```python
from build123d import *

# Parameters (mm, degrees)
SKETCH1_R               = 0.8
BOSS_EXTRUDE1_DEPTH     = 0.75
SKETCH2_R               = 0.8
BOSS_EXTRUDE2_DEPTH     = 2.5
CHAMFER1_SIZE           = 1.625
CUT_EXTRUDE1_DEPTH      = 24.451236904
CUT_EXTRUDE1_DEPTH_BACK = 24.451236904
SKETCH3_W               = 10.5
SKETCH3_H               = 2


with BuildPart() as part:
    # Sketch1 → Boss-Extrude1 (new, symmetric)
    with BuildSketch(Plane(origin=(0, 0, 0), x_dir=(1, 0, 0), z_dir=(0, 1, 0))):
        with BuildLine():
            ThreePointArc((1.600460999, 1.920553199), (-1.920553199, 1.600460999), (-1.600460999, -1.920553199))
            ThreePointArc((-1.600460999, -1.920553199), (10, -6.120499352), (21.600460999, -1.920553199))
            ThreePointArc((21.600460999, -1.920553199), (21.920553199, 1.600460999), (18.399539001, 1.920553199))
            ThreePointArc((18.399539001, 1.920553199), (10, -1.120499352), (1.600460999, 1.920553199))
        make_face()
        with Locations(Location((0, 0, 0), (0, 0, 270))):
            Circle(SKETCH1_R, mode=Mode.SUBTRACT)
        with Locations(Location((20, 0, 0), (0, 0, 270))):
            Circle(SKETCH1_R, mode=Mode.SUBTRACT)
    extrude(amount=BOSS_EXTRUDE1_DEPTH, both=True)

    # Sketch2 → Boss-Extrude2 (add, symmetric)
    with BuildSketch(Plane(origin=(0, 0, 0), x_dir=(1, 0, 0), z_dir=(0, 1, 0))):
        with BuildLine():
            Line((10, -1.120499352), (10, -6.120499352))
            ThreePointArc((10, -6.120499352), (16.168675771, -5.038190514), (21.600460999, -1.920553199))
            ThreePointArc((21.600460999, -1.920553199), (21.920553199, 1.600460999), (18.399539001, 1.920553199))
            ThreePointArc((18.399539001, 1.920553199), (14.466549452, -0.336832626), (10, -1.120499352))
        make_face()
        with Locations(Location((20, 0, 0), (0, 0, 270))):
            Circle(SKETCH2_R, mode=Mode.SUBTRACT)
    extrude(amount=BOSS_EXTRUDE2_DEPTH, both=True)

    # Chamfer1
    chamfer1_edges = [part.edges().sort_by_distance(p)[0] for p in [
        (10, -2.5, 3.620499352),
        (10, 2.5, 3.620499352),
    ]]
    chamfer(chamfer1_edges, length=CHAMFER1_SIZE)

    # Sketch3 → Cut-Extrude1 (cut, two sides: drawn at the far end of the back side and taken through both)
    with BuildSketch(Plane(origin=(0, 0, 0), x_dir=(-1, 0, 0), z_dir=(0, 0, -1)).offset(-CUT_EXTRUDE1_DEPTH_BACK)):
        with Locations((-17.25, 0)):
            Rectangle(SKETCH3_W, SKETCH3_H)
    extrude(amount=CUT_EXTRUDE1_DEPTH + CUT_EXTRUDE1_DEPTH_BACK, mode=Mode.SUBTRACT)


solid = part.part
```
Check sheet for the modelled part. Datum: model origin and axes. Units: mm. A direction names the side the tool comes from. Coordinates: 2 decimals unless noted, no trailing zeros. Order: outer loops, then holes, each group sorted by start corner. A loop starts at its lowest first (then second) coordinate and runs counter-clockwise, first axis right, second up. Notation, with made-up numbers: (11, 45) -> (38, 45) arc R22 cw to (38, 83) -> close; hole circle Ø2 at (-9.5, -8). An arc over 180 degrees is marked (long way). Write item = value, one per line. Start each with the question number.
1) Cross-section at D-D (z = 4). Enter the section's corners in (x, y) (3 decimals), then the cut area to 3 significant figures.
2) Cross-section at C-C (z = 0). Enter the section's corners in (x, y).
3) Mould release check, pull along Z, two halves, no side actions. Record for faces 6 (the cylindrical face through (-1.885, 0.01, -1.642)), 7 (the flat face through (10.824, -1.699, 3.534)), 8 (the cylindrical face through (-0.49, -0.01, -0.63)), 9 (the cylindrical face through (19.29, 1.74, 0.37)): +Z half, -Z half, draft (parallel to the pull), parting line (faces both ways), or undercut.
4) Cross-section at B-B (x = 17). Enter the section's corners in (y, z).
5) Cross-section at A-A (y = 0.25). Enter the section's corners in (x, z).
6) Go/stop test with flat-tipped pins: P1, Ø1.6, axis at y = 0, z = 2.5, coming from the +X side; P2, Ø1.5, axis at x = 15, y = 1.5, coming from the -Z side; P3, Ø4, axis at x = 7.5, z = 4.5, coming from the +Y side. Record where each tip stops, or that it passes through.
7) Access from +Z, -Z, +X, -X, +Y, -Y to the whole of each face (thin tool, end or side, straight path). Record for faces 1 (the flat face through (17, 2.5, 2)), 2 (the flat face through (4, 0.75, 2)), 3 (the cylindrical face through (19.29, -1.76, 0.37)), 4 (the flat face through (4, -0.75, 2)), 5 (the flat face through (17, 1, 2)).
8) Material ranges on L1, parallel to Y at x = 12.75, z = 3.5; L2, parallel to X at y = -2.2, z = -0.5; L3, parallel to Y at x = 3, z = 2.25, recorded low to high.
Ans:
q1.outline = (1.494, -0.75) -> (10, -0.75) -> (10, -0.875) -> (11.625, -2.5) -> (18.506, -2.5) -> (18.506, -1) -> (12, -1) -> (12, 1) -> (18.506, 1) -> (18.506, 2.5) -> (11.625, 2.5) -> (10, 0.875) -> (10, 0.75) -> (1.494, 0.75) -> close
q1.area = 39.6 mm²
q2.outline = (-2.5, -0.75) -> (-0.8, -0.75) -> (-0.8, 0.75) -> (-2.5, 0.75) -> close; (0.8, -0.75) -> (4.69, -0.75) -> (4.69, 0.75) -> (0.8, 0.75) -> close; (15.31, -2.5) -> (19.2, -2.5) -> (19.2, -1) -> (15.31, -1) -> close; (15.31, 1) -> (19.2, 1) -> (19.2, 2.5) -> (15.31, 2.5) -> close; (20.8, -2.5) -> (22.5, -2.5) -> (22.5, -1) -> (20.8, -1) -> close; (20.8, 1) -> (22.5, 1) -> (22.5, 2.5) -> (20.8, 2.5) -> close
q3.face_6 = parting line
q3.face_7 = draft
q3.face_8 = undercut
q3.face_9 = undercut
q4.outline = (-2.5, -0.9) -> (-1, -0.9) -> (-1, 4.71) -> (-2.5, 4.71) -> close; (1, -0.9) -> (2.5, -0.9) -> (2.5, 4.71) -> (1, 4.71) -> close
q5.outline = (-1.6, 1.92) arc R2.5 ccw to (1.6, -1.92) arc R13.12 cw to (12, 0.97) -> (12, 6.01) arc R18.12 ccw to start; hole circle Ø1.6 at (0, 0)
q6.P1 = 12
q6.P2 = -0.21
q6.P3 = 0.75
q7.face_1 = +Z, -Z, +X, -X, +Y
q7.face_2 = +Z, -Z, -X, +Y
q7.face_3 = +Y, -Y
q7.face_4 = +Z, -Z, -X, -Y
q7.face_5 = +Z, -Z, +X
q8.L1 = -2.5 to -1, 1 to 2.5
q8.L2 = 16.32 to 19.38, 20.62 to 22.45
q8.L3 = -0.75 to 0.75
